Geometry check sheet. Reference: the model listing, model coordinates, mm. Face numbers are marked on the shaded views. A direction names the side the tool comes from. Give positions to 0.01 mm unless a question says otherwise; leave off trailing zeros. Order: outer loops, then holes, each group sorted by start corner. A loop starts at its lowest first (then second) coordinate and runs counter-clockwise, first axis right, second up. Notation, with made-up numbers: M -10.5,82.5 L 36.5,82.5 A10 cw 36.5,87.5 Z; hole C 3.25,14 d3. An arc over 180 degrees is marked long. Put each result on its own line as item: value. Start each with the question number.
Q1. Section check D-D on z = -8.5. Record the cut outline in (x, y).
Q2. Section check C-C on z = -2.5. Record the cut outline in (x, y).
Q3. Mould release check, pull along X, two halves, no side actions. Record for the marked faces 3, 4 and 5: +X half, -X half, draft (parallel to the pull), parting line (faces both ways), or undercut.
Q4. Material ranges on L1, parallel to Y at x = 0, z = 7.5; L2, parallel to X at y = 2, z = -8.5; L3, parallel to X at y = 2.25, z = -3.5, recorded low to high.
Q5. Section check A-A on y = 4.75. Record the cut outline in (x, z).
Q6. Section check B-B on x = 0. Record the cut outline in (y, z), then the cut area to 3 significant figures.
Q7. Go/stop test with flat-tipped pins: pin 1 (2 mm diameter, centred on y = 4, z = -7.5, fed in from -X); pin 2 (5.5 mm diameter, centred on x = 5, z = 3.5, fed in from +Y). Record where each tip stops, or that it passes through.
Q8. Access from +Z, -Z, +X, -X, +Y, -Y to the whole of each face (thin tool, end or side, straight path). Record for the marked faces 1 and 2.
Autodesk Inventor part; units mm, degrees
ref_plane "YZ Plane" through (0, 0, 0) normal (1, 0, 0) x (0, 1, 0)
ref_plane "XZ Plane" through (0, 0, 0) normal (0, 1, 0) x (-1, 0, 0)
ref_plane "XY Plane" through (0, 0, 0) normal (0, 0, 1) x (1, 0, 0)
sketch "Sketch1" plane through (0, 0, 0) normal (0, 1, 0) x (-1, 0, 0)
  circle A0 centre (0, 0) radius 4.1
  circle A1 centre (0, 0) radius 11
  dimension "d0" = 8.2
  dimension "d1" = 22
extrude "Extrusion1" add sketch "Sketch1" along normal blind 4
sketch "Sketch2" plane through (0, 4, 0) normal (0, 1, 0) x (1, 0, 0)
  line L0 (0, 0) -> (-8.1688, -0.7147) construction
  line L1 (0, 0) -> (-8.1688, 0.7147) construction
  arc A0 (-4.0844, 0.3573) -> (-4.0844, -0.3573) centre (10.5368, 0) ccw
  line L2 (-4.0844, 0.3573) -> (-10.9581, 0.9587)
  line L3 (-15.4, 0) -> (15.4, 0) construction
  circle A1 centre (0, 0) radius 4.1 construction
  circle A2 centre (0, 0) radius 11 construction
  line L4 (-4.0844, -0.3573) -> (-10.9581, -0.9587)
  circle A3 centre (0, 0) radius 11
  dimension "d4" = 10
extrude "Extrusion2" add sketch "Sketch2" along normal blind 2 contours A0 L4 A3 L2 picked at (-8.693, 0.0397)
sketch "Sketch3" plane through (0, 0, 0) normal (0, 0, 1) x (1, 0, 0)
  circle A0 centre (0, 2) radius 1.25
  line L0 (11, 0) -> (-11, 0)
  point P0 (0, 0)
  dimension "d7" = 2.5
  dimension "d8" = 2
extrude "Extrusion3" cut sketch "Sketch3" against normal through all both and the other way through all
pattern_circular "Circular Pattern1" count 2 over 360 about axis through (0, -10, 0) along (0, 1, 0) of "Extrusion2"
properties part number "170d_coupler"
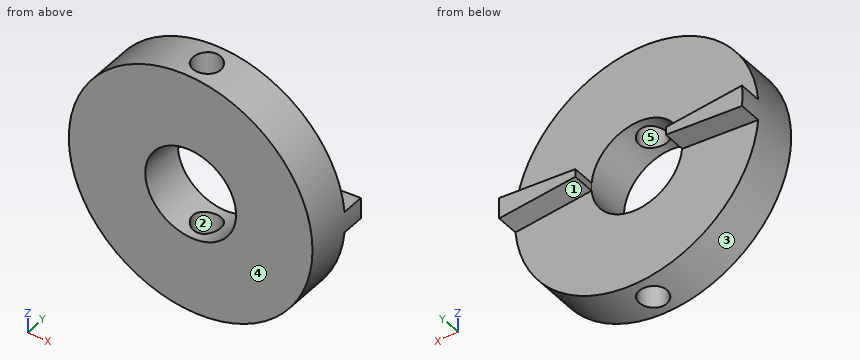
Results found:
1. outline: M -6.98,0 L 6.98,0 L 6.98,4 L -6.98,4 Z; hole C 0,2 d2.5
2. outline: M -10.71,0 L -3.25,0 L -3.25,4 L -10.71,4 Z; M 3.25,0 L 10.71,0 L 10.71,4 L 3.25,4 Z
3. face 3: parting line
3. face 4: draft
3. face 5: undercut
4. L1: y = 0 to 0.75, 3.25 to 4
4. L2: x = -6.98 to -1.25, 1.25 to 6.98
4. L3: x = -10.43 to -2.14, 2.14 to 10.43
5. outline: M -10.96,-0.96 L -4.08,-0.36 A14.63 cw -4.08,0.36 L -10.96,0.96 A11 ccw Z; M 4.08,-0.36 L 10.96,-0.96 A11 ccw 10.96,0.96 L 4.08,0.36 A14.63 cw Z
6. outline: M 0,-11 L 0.75,-11 L 0.75,-4.1 L 0,-4.1 Z; M 0,4.1 L 0.75,4.1 L 0.75,11 L 0,11 Z; M 3.25,-11 L 4,-11 L 4,-4.1 L 3.25,-4.1 Z; M 3.25,4.1 L 4,4.1 L 4,11 L 3.25,11 Z
6. area: 20.7 mm^2
7. pin 1: stops at x = -8.87
7. pin 2: stops at y = 4
8. face 1: -Z, +Y
8. face 2: +Z, -Z
